from build123d import *

# Parameters (mm, degrees)
SKETCH_1_R          = 31.5
EXTRUDE_1_DEPTH     = 6
SKETCH_2_R          = 15
EXTRUDE_2_DEPTH     = 50
SKETCH_3_R          = 2.6
CUT_EXTRUDE_1_DEPTH = 72.557669051


with BuildPart() as part:
    # 草图1 → 凸台-拉伸1 (new body)
    with BuildSketch(Plane(origin=(0, 0, 0), x_dir=(1, 0, 0), z_dir=(0, 1, 0))):
        with Locations(Location((0, 0, 0), (0, 0, 270))):
            Circle(SKETCH_1_R)
    extrude(amount=EXTRUDE_1_DEPTH)

    # 草图2 → 凸台-拉伸2 (add)
    with BuildSketch(Plane(origin=(0, 6, 0), x_dir=(1, 0, 0), z_dir=(0, 1, 0))):
        with Locations(Location((0, 0, 0), (0, 0, 270))):
            Circle(SKETCH_2_R)
    extrude(amount=EXTRUDE_2_DEPTH)

    # 草图3 → 切除-拉伸1 (cut, through all)
    with BuildSketch(Plane.XZ):
        with Locations(Location((-21.650635095, -12.5, 0), (0, 0, 270))):
            Circle(SKETCH_3_R)
        with Locations(Location((0, 25, 0), (0, 0, 270))):
            Circle(SKETCH_3_R)
        with Locations(Location((21.650635095, -12.5, 0), (0, 0, 270))):
            Circle(SKETCH_3_R)
    extrude(amount=-CUT_EXTRUDE_1_DEPTH, mode=Mode.SUBTRACT)


solid = part.part
Design review of the part built by this model. Coordinates are the model's own, in mm. Give positions to 0.01 mm unless a question says otherwise; leave off trailing zeros. Order: outer loops, then holes, each group sorted by start corner. A loop starts at its lowest first (then second) coordinate and runs counter-clockwise, first axis right, second up.
1. To check wall thickness, follow L1, parallel to Y at x = 18.5, z = -9.5; L2, parallel to Z at x = 0.5, y = 51; L3, parallel to X at y = 2, z = 25. State the ranges of each line that lie inside material, in increasing order.
Solution:
L1: y = 0 to 6
L2: z = -14.99 to 14.99
L3: x = -19.16 to -2.6, 2.6 to 19.16
2. Add section C-C, the plane x = 10. State the section outline as (y, z) points.
Solution:
outline: (0, -29.87) - (6, -29.87) - (6, -11.18) - (56, -11.18) - (56, 11.18) - (6, 11.18) - (6, 29.87) - (0, 29.87) - close
3. Mouldability with a two-part tool opening along Z and no side actions: class faces 1 (the cylindrical face through (0.66, 30.65, -14.985)), 2 (the cylindrical face through (-20.87, 2.96, -14.98)), 3 (the flat face through (-7, 6, 14)), 4 (the cylindrical face through (0.78, 2.96, 22.52)) as +Z half, -Z half, draft (parallel to the pull), parting line (faces both ways), or undercut.
Solution:
face 1: parting line
face 2: undercut
face 3: draft
face 4: undercut
4. Add section B-B, the plane z = -13. State the section outline as (x, y) points, then the cut area to 3 significant figures.
Solution:
outline: (-28.69, 0) - (-24.2, 0) - (-24.2, 6) - (-28.69, 6) - close; (-19.1, 0) - (19.1, 0) - (19.1, 6) - (7.48, 6) - (7.48, 56) - (-7.48, 56) - (-7.48, 6) - (-19.1, 6) - close; (24.2, 0) - (28.69, 0) - (28.69, 6) - (24.2, 6) - close
area: 1,030 mm2
5. Add section A-A, the plane z = 25. State the section outline as (x, y) points, then the cut area to 3 significant figures.
Solution:
outline: (-19.16, 0) - (-2.6, 0) - (-2.6, 6) - (-19.16, 6) - close; (2.6, 0) - (19.16, 0) - (19.16, 6) - (2.6, 6) - close
area: 199 mm2
6. Add section D-D, the plane z = 0. State the section outline as (x, y) points, then the cut area to 3 significant figures.
Solution:
outline: (-31.5, 0) - (31.5, 0) - (31.5, 6) - (15, 6) - (15, 56) - (-15, 56) - (-15, 6) - (-31.5, 6) - close
area: 1,880 mm2
7. For pin 1 Ø6 at (x, z) = (-21.65, -12.5) entering from -Y; pin 2 Ø3 at (y, z) = (47, -6) entering from -X; pin 3 Ø6 at (x, y) = (2.5, 29.5) entering from +Z; pin 4 Ø8 at (x, y) = (16.5, 39) entering from -Z, all flat-tipped, find the tip position at first contact; note any pin that passes through.
Solution:
pin 1: stops at y = 0
pin 2: stops at x = -14.31
pin 3: stops at z = 15
pin 4: stops at z = -8.29
